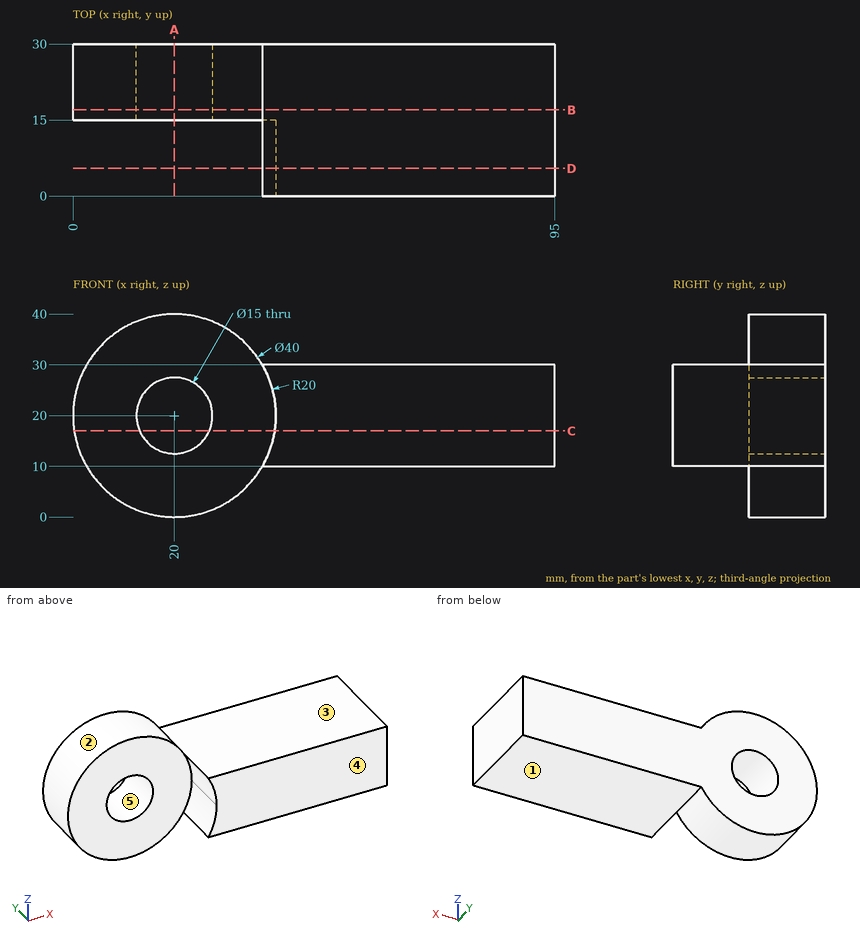
Drawing for the job (mm, zero at the part's lowest x, y, z). A direction names the side the tool comes from. Round coordinates to 2 decimals unless told otherwise and drop trailing zeros. Loops run counter-clockwise (first coordinate to the right, second up) from the corner with the lowest first, then second, coordinate; pieces in that order, holes last. Notation, with made-up numbers: M 1.25,68.25 L 59.25,68.25 A28 cw 59.25,87.25 Z; hole C 60.25,21 d2. An arc over 180 degrees is marked long. Use a Markdown table: item, result. Add a question column.
(1) Cut at D-D (y = 5.5). Give the cut face in (x, z), and give its area (3 significant figures).
(2) Cut at A-A (x = 20). Give the cut face in (y, z).
(3) Which spindle directions (+Z, -Z, +X, -X, +Y, -Y) get a long thin tool onto all of the face, cutting with end or side? Do the marked faces 1 and 2. Say none if no direction does.
(4) Flat gauge pins, fed straight in: pin 1 (1.5 mm diameter, centred on x = 67.5, y = 13, fed in from -Z); pin 2 (1.5 mm diameter, centred on x = 16, y = 16.5, fed in from -Z); pin 3 (17 mm diameter, centred on x = 20, z = 20, fed in from -Y). Where does each tip first touch, or does it go through?
(5) Cut at B-B (y = 17). Give the cut face in (x, z), and give its area (3 significant figures).
(6) Drill centre lines: line 1 (Z direction, x = 20, y = 23); line 2 (X direction, y = 20.5, z = 20); line 3 (Z direction, x = 79.5, y = 24.75). Where is each one in solid material? Low to high.
(7) Cut at C-C (z = 17). Give the cut face in (x, y).
(8) Pull direction Z, two halves, no side cores. Call the marked faces 3, 4 and 5: +Z half, -Z half, draft (parallel to the pull), parting line (faces both ways), or undercut.
Geometry says:
| question | item | result |
|---|---|---|
| 1 | outline | M 37.32,10 L 95,10 L 95,30 L 37.32,30 A20 cw 40,20 A20 cw Z |
| 1 | area | 1,120 mm² |
| 2 | outline | M 15,0 L 30,0 L 30,12.5 L 15,12.5 Z; M 15,27.5 L 30,27.5 L 30,40 L 15,40 Z |
| 3 | face 1 | -Z, +X, +Y, -Y |
| 3 | face 2 | +Y, -Y |
| 4 | pin 1 | stops at z = 10 |
| 4 | pin 2 | stops at z = 0.27 |
| 4 | pin 3 | stops at y = 15 |
| 5 | outline | M 37.32,10 L 95,10 L 95,30 L 37.32,30 A20 ccw long Z; hole C 20,20 d15 |
| 5 | area | 2,200 mm² |
| 6 | line 1 | z = 0 to 12.5, 27.5 to 40 |
| 6 | line 2 | x = 0 to 12.5, 27.5 to 95 |
| 6 | line 3 | z = 10 to 30 |
| 7 | outline | M 0.23,15 L 13.13,15 L 13.13,30 L 0.23,30 Z; M 26.87,15 L 39.77,15 L 39.77,0 L 95,0 L 95,30 L 26.87,30 Z |
| 8 | face 3 | +Z half |
| 8 | face 4 | draft |
| 8 | face 5 | undercut |
